Check sheet for the modelled part. Datum: model origin and axes. Units: mm. A direction names the side the tool comes from. Give positions to 0.01 mm unless a question says otherwise; leave off trailing zeros. Order: outer loops, then holes, each group sorted by start corner. A loop starts at its lowest first (then second) coordinate and runs counter-clockwise, first axis right, second up. Notation, with made-up numbers: (47.5, -9) -> (91.5, -9) arc R5 cw to (91.5, -1) -> close; hole circle Ø11 at (11, -36). An arc over 180 degrees is marked (long way). One line per question, with ' | ' between items.
```python
from build123d import *

# Parameters (mm, degrees)
SKETCH1_W           = 6
SKETCH1_H           = 6
BOSS_EXTRUDE1_DEPTH = 15
SKETCH3_W           = 10
SKETCH3_H           = 45
BOSS_EXTRUDE2_DEPTH = 2
SKETCH4_W           = 4
SKETCH4_H           = 5
BOSS_EXTRUDE3_DEPTH = 2
SKETCH5_W           = 4
SKETCH5_H           = 5
BOSS_EXTRUDE4_DEPTH = 2
SKETCH6_W           = 4
SKETCH6_H           = 3
BOSS_EXTRUDE5_DEPTH = 3
SKETCH7_W           = 4
SKETCH7_H           = 3
BOSS_EXTRUDE6_DEPTH = 3
SKETCH8_R           = 2.5
CUT_EXTRUDE1_DEPTH  = 1
SKETCH9_R           = 2.5
BOSS_EXTRUDE7_DEPTH = 25


with BuildPart() as part:
    # Sketch1 → Boss-Extrude1 (new body)
    with BuildSketch(Plane(origin=(0, 0, 0), x_dir=(1, 0, 0), z_dir=(0, 1, 0))):
        Rectangle(SKETCH1_W, SKETCH1_H)
    extrude(amount=BOSS_EXTRUDE1_DEPTH)

    # Sketch3 → Boss-Extrude2 (add)
    with BuildSketch(Plane(origin=(0, 0, 0), x_dir=(1, 0, 0), z_dir=(0, 1, 0))):
        with Locations((-0.682406889, -13.428719973)):
            Rectangle(SKETCH3_W, SKETCH3_H)
    extrude(amount=-BOSS_EXTRUDE2_DEPTH)

    # Sketch4 → Boss-Extrude3 (add)
    with BuildSketch(Plane.XY.offset(35.928719973)):
        with Locations((-0.302179452, -4.5)):
            Rectangle(SKETCH4_W, SKETCH4_H)
    extrude(amount=-BOSS_EXTRUDE3_DEPTH)

    # Sketch5 → Boss-Extrude4 (add)
    with BuildSketch(Plane(origin=(0, 0, -9.071280027), x_dir=(-1, 0, 0), z_dir=(0, 0, -1))):
        with Locations((0.302179452, -4.5)):
            Rectangle(SKETCH5_W, SKETCH5_H)
    extrude(amount=-BOSS_EXTRUDE4_DEPTH)

    # Sketch6 → Boss-Extrude5 (add)
    with BuildSketch(Plane(origin=(0, 0, 33.928719973), x_dir=(-1, 0, 0), z_dir=(0, 0, -1))):
        with Locations((0.302179452, -5.5)):
            Rectangle(SKETCH6_W, SKETCH6_H)
    extrude(amount=BOSS_EXTRUDE5_DEPTH)

    # Sketch7 → Boss-Extrude6 (add)
    with BuildSketch(Plane.XY.offset(-7.071280027)):
        with Locations((-0.302179452, -5.5)):
            Rectangle(SKETCH7_W, SKETCH7_H)
    extrude(amount=BOSS_EXTRUDE6_DEPTH)

    # Sketch8 → Cut-Extrude1 (cut)
    with BuildSketch(Plane.XY.offset(3)):
        with Locations((0, 10.46201193)):
            Circle(SKETCH8_R)
    extrude(amount=-CUT_EXTRUDE1_DEPTH, mode=Mode.SUBTRACT)

    # Sketch9 → Boss-Extrude7 (add)
    with BuildSketch(Plane.XY.offset(2)):
        with Locations((0, 10.44523286)):
            Circle(SKETCH9_R)
    extrude(amount=BOSS_EXTRUDE7_DEPTH)


solid = part.part
```
Q1. Mould release check, pull along Z, two halves, no side actions. Record for faces 1 (the face through (-1, -3, 35.929)), 2 (the face through (-5.682, -1, 14)), 3 (the face through (0, -4, 32)): pulls with the +Z half, pulls with the -Z half, needs draft (parallel to the pull), parting line crosses it, or undercut.
Result sheet:
face 1: pulls with the +Z half | face 2: needs draft | face 3: undercut
Q2. Depth check by flat-ended pin: pin 1 Ø3 at (x, y) = (-3, 6) entering from -Z; pin 2 Ø5.5 at (y, z) = (-5, -6.5) entering from -X; pin 3 Ø2 at (x, z) = (1.5, 13) entering from +Y. Enter the tip coordinate at first touch or a pass-through.
Result sheet:
pin 1: stops at z = -3 | pin 2: stops at x = -2.3 | pin 3: stops at y = 12.89
Q3. Section check B-B (y = -4.5). Enter the section's corners in (x, z), and give its area (3 significant figures).
Result sheet:
outline: (-2.3, -9.07) -> (1.7, -9.07) -> (1.7, -4.07) -> (-2.3, -4.07) -> close; (-2.3, 30.93) -> (1.7, 30.93) -> (1.7, 35.93) -> (-2.3, 35.93) -> close | area: 40.0 mm2
Q4. Thickness scan on line 1 (Y direction, x = 0, z = 17.5); line 2 (Z direction, x = -2, y = -6); line 3 (Y direction, x = -4.5, z = 21.5). Record the ranges inside material, lowest first.
Result sheet:
line 1: y = -2 to 0, 7.95 to 12.95 | line 2: z = -9.07 to -4.07, 30.93 to 35.93 | line 3: y = -2 to 0
Q5. Section check A-A (z = -6). Enter the section's corners in (x, y), and give its area (3 significant figures).
Result sheet:
outline: (-5.68, -2) -> (4.32, -2) -> (4.32, 0) -> (-5.68, 0) -> close; (-2.3, -7) -> (1.7, -7) -> (1.7, -4) -> (-2.3, -4) -> close | area: 32.0 mm2
Q6. Section check C-C (z = -1.5). Enter the section's corners in (x, y).
Result sheet:
outline: (-5.68, -2) -> (4.32, -2) -> (4.32, 0) -> (3, 0) -> (3, 15) -> (-3, 15) -> (-3, 0) -> (-5.68, 0) -> close
Q7. Access from +Z, -Z, +X, -X, +Y, -Y to the whole of each face (thin tool, end or side, straight path). Record for faces 4 (the face through (-2.302, -5, -7)), 5 (the face through (0, 10, 27)), 6 (the face through (3, 7, 0)).
Result sheet:
face 4: +Z, -Z, -X, -Y | face 5: +Z, +X, -X, +Y | face 6: +Z, -Z, +X, +Y
